```python
from build123d import *

# Parameters (mm, degrees)
SKETCH1_R           = 26
BOSS_EXTRUDE1_DEPTH = 38
SKETCH2_R           = 3.5
CUT_EXTRUDE1_DEPTH  = 117.250849889


with BuildPart() as part:
    # Sketch1 → Boss-Extrude1 (new body)
    with BuildSketch(Plane(origin=(0, 0, 0), x_dir=(1, 0, 0), z_dir=(0, 1, 0))):
        Polygon((88.75, 0), (90, 0), (90, 18.75), (88.75, 20), (88.75, 52), (73.75, 52), (62.74, 63.01), (27.26, 63.01), (16.25, 52), (1.25, 52), (1.25, 20), (0, 18.75), (0, 0), (1.25, 0), (45, 0), align=None)
        with Locations(Location((45, 33, 0), (0, 0, 270))):
            Circle(SKETCH1_R, mode=Mode.SUBTRACT)
    extrude(amount=BOSS_EXTRUDE1_DEPTH)

    # Sketch2 → Cut-Extrude1 (cut, through all)
    with BuildSketch(Plane.XY):
        with Locations((10, 28)):
            Circle(SKETCH2_R)
        with Locations((10, 10)):
            Circle(SKETCH2_R)
        with Locations((80, 28)):
            Circle(SKETCH2_R)
        with Locations((80, 10)):
            Circle(SKETCH2_R)
    extrude(amount=-CUT_EXTRUDE1_DEPTH, mode=Mode.SUBTRACT)


solid = part.part
```
Verification items for the finished model (mm, model axes). A direction names the side the tool comes from. Coordinates: 2 decimals unless noted, no trailing zeros. Loops run counter-clockwise (first coordinate to the right, second up) from the corner with the lowest first, then second, coordinate; pieces in that order, holes last. Notation, with made-up numbers: (-36.75, 49) -> (14.25, 49) arc R5 ccw to (14.25, 53) -> close; hole circle Ø11 at (-19.75, 25.25). An arc over 180 degrees is marked (long way). Put each result on its own line as item: value.
1. Section check A-A, the plane z = -33. Record the boundary of the cut face in (x, y), then the cut area to 3 significant figures.
Result set:
outline: (1.25, 0) -> (19, 0) -> (19, 38) -> (1.25, 38) -> close; (71, 0) -> (88.75, 0) -> (88.75, 38) -> (71, 38) -> close; hole circle Ø7 at (10, 10); hole circle Ø7 at (10, 28); hole circle Ø7 at (80, 10); hole circle Ø7 at (80, 28)
area: 1,200 mm^2
2. Section check C-C, the plane x = 80. Record the boundary of the cut face in (y, z).
Result set:
outline: (0, -52) -> (6.5, -52) -> (6.5, 0) -> (0, 0) -> close; (13.5, -52) -> (24.5, -52) -> (24.5, 0) -> (13.5, 0) -> close; (31.5, -52) -> (38, -52) -> (38, 0) -> (31.5, 0) -> close
3. Mould release check, pull along Y, two halves, no side actions. Record for faces 1 (the face through (1.25, 19, -36)), 2 (the face through (9.54, 31.47, -25.64)), 3 (the face through (44, 0, -4)): pulls with the +Y half, pulls with the -Y half, needs draft (parallel to the pull), parting line crosses it, or undercut.
Result set:
face 1: needs draft
face 2: undercut
face 3: pulls with the -Y half
4. Tool access check on faces 4 (the face through (9, 19, -52)), 5 (the face through (88.75, 19, -36)), 6 (the face through (7.2, 7.9, -25.6)). Record the directions out of +Z, -Z, +X, -X, +Y, -Y that give a thin tool (end or side, any length) a straight path to the whole face; none if there is none.
Result set:
face 4: -Z, -X, +Y, -Y
face 5: -Z, +X, +Y, -Y
face 6: +Z, -Z
5. Thickness scan on line 1 (Y direction, x = 10, z = -18); line 2 (Z direction, x = 46, y = 32); line 3 (X direction, y = 27.5, z = -33). Record the ranges inside material, lowest first.
Result set:
line 1: y = 0 to 6.5, 13.5 to 24.5, 31.5 to 38
line 2: z = -63.01 to -58.98, -7.02 to 0
line 3: x = 1.25 to 6.54, 13.46 to 19, 71 to 76.54, 83.46 to 88.75
6. Section check B-B, the plane y = 10. Record the boundary of the cut face in (x, z).
Result set:
outline: (0, -18.75) -> (1.25, -20) -> (1.25, -52) -> (6.5, -52) -> (6.5, 0) -> (0, 0) -> close; (13.5, -52) -> (16.25, -52) -> (27.26, -63.01) -> (62.74, -63.01) -> (73.75, -52) -> (76.5, -52) -> (76.5, 0) -> (13.5, 0) -> close; (83.5, -52) -> (88.75, -52) -> (88.75, -20) -> (90, -18.75) -> (90, 0) -> (83.5, 0) -> close; hole circle Ø52 at (45, -33)
7. Section check D-D, the plane x = 45. Record the boundary of the cut face in (y, z).
Result set:
outline: (0, -63.01) -> (38, -63.01) -> (38, -59) -> (0, -59) -> close; (0, -7) -> (38, -7) -> (38, 0) -> (0, 0) -> close
8. Gauge pin test, flat ends, axial feed: P1, Ø16, axis at y = 26, z = -33.5, coming from the +X side; P2, Ø5.5, axis at x = 10, y = 10, coming from the -Z side (1 decimal); P3, Ø12, axis at x = 5, y = 12.5, coming from the -Z side; P4, Ø6, axis at y = 22.5, z = -43, coming from the -X side. Record the tip position at first contact, or that the pin passes through.
Result set:
P1: stops at x = 88.75
P2: passes through
P3: stops at z = -52
P4: stops at x = 1.25
